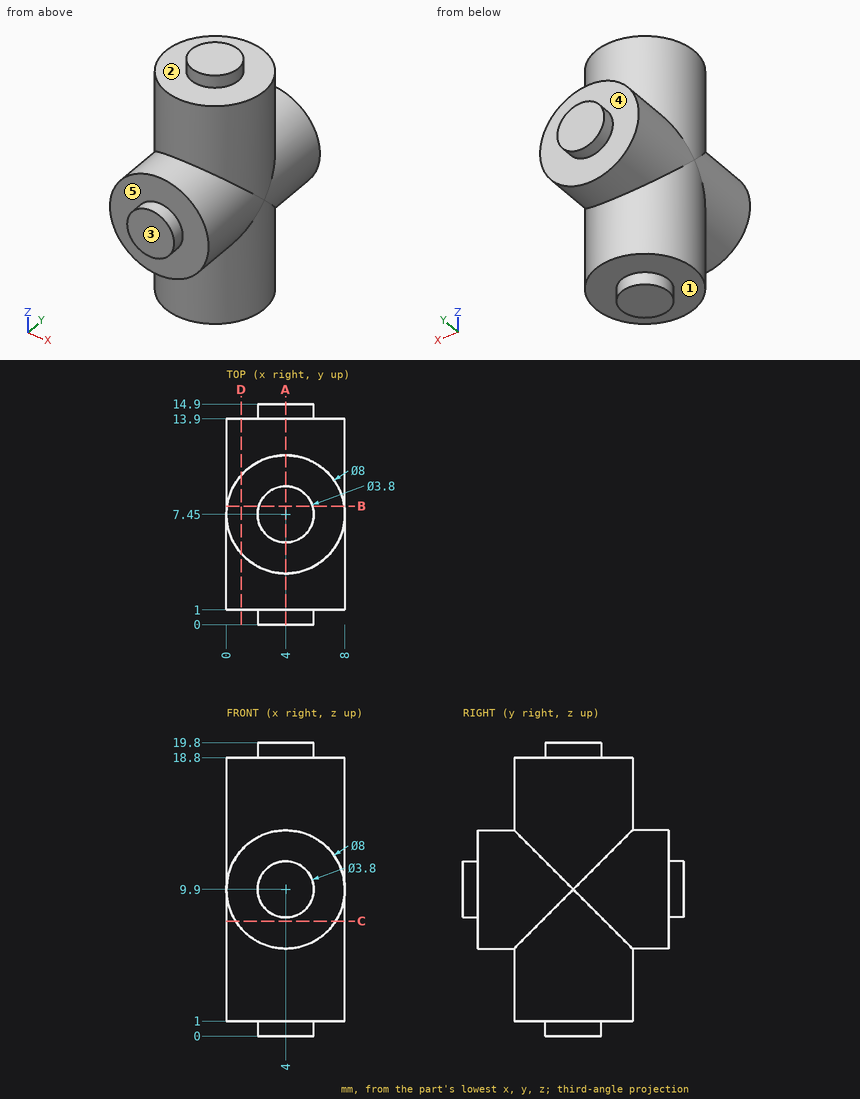
Could you check a few things on this drawing? It's one solid part, dimensions in mm from its lowest x, y, z. A direction names the side the tool comes from. Coordinates: 2 decimals unless noted, no trailing zeros. Order: outer loops, then holes, each group sorted by start corner. A loop starts at its lowest first (then second) coordinate and runs counter-clockwise, first axis right, second up. Notation, with made-up numbers: (-9, 28) - (13, 28) arc R24 cw to (13, 60) - close; hole circle Ø9 at (-12.75, 88). An arc over 180 degrees is marked (long way). Answer as a JSON object with one key per item and string values. Group by question number.
Q1. Imagine slicing it at A-A (x = 4). Please give me the cut outline in (y, z), and give its area (3 significant figures).
Q2. Imagine slicing it at B-B (y = 8). Please give me the cut outline in (x, z).
Q3. Imagine slicing it at D-D (x = 1). Please give me the cut outline in (y, z), and give its area (3 significant figures).
Q4. Imagine slicing it at C-C (z = 7.75). Please give me the cut outline in (x, y).
Q5. I need wall thicknesses on line 1 (Y direction, x = 2, z = 13); line 2 (Z direction, x = 7.25, y = 7.25); line 3 (Y direction, x = 4.25, z = 19). Which ranges of each line are inside material? Lowest first, please. Write a range as from..to.
Q6. On a 3-axis mill with a long thin cutter (end or side, diameter ignored), from which of +Z, -Z, +X, -X, +Y, -Y can I reach the whole of each face in a straight line? I mean the marked faces 1, 2, 3, 4 and 5. Say none if no direction works.
Q7. Will these pins go through, and if not, where does the flat tip stop? P1, Ø1, axis at x = 4, z = 16, coming from the -Y side; P2, Ø4, axis at x = 2.5, y = 13, coming from the +Z side; P3, Ø4, axis at y = 12, z = 17.5, coming from the -X side.
Determined:
{
 "1": {"outline": "(0, 8) - (1, 8) - (1, 5.9) - (3.45, 5.9) - (3.45, 1) - (5.55, 1) - (5.55, 0) - (9.35, 0) - (9.35, 1) - (11.45, 1) - (11.45, 5.9) - (13.9, 5.9) - (13.9, 8) - (14.9, 8) - (14.9, 11.8) - (13.9, 11.8) - (13.9, 13.9) - (11.45, 13.9) - (11.45, 18.8) - (9.35, 18.8) - (9.35, 19.8) - (5.55, 19.8) - (5.55, 18.8) - (3.45, 18.8) - (3.45, 13.9) - (1, 13.9) - (1, 11.8) - (0, 11.8) - close", "area": "197 mm2"},
 "2": {"outline": "(0.04, 1) - (2.18, 1) - (2.18, 0) - (5.82, 0) - (5.82, 1) - (7.96, 1) - (7.96, 9.35) arc R4 ccw to (7.96, 10.45) - (7.96, 18.8) - (5.82, 18.8) - (5.82, 19.8) - (2.18, 19.8) - (2.18, 18.8) - (0.04, 18.8) - (0.04, 10.45) arc R4 ccw to (0.04, 9.35) - close"},
 "3": {"outline": "(1, 7.25) - (4.8, 7.25) - (4.8, 1) - (10.1, 1) - (10.1, 7.25) - (13.9, 7.25) - (13.9, 12.55) - (10.1, 12.55) - (10.1, 18.8) - (4.8, 18.8) - (4.8, 12.55) - (1, 12.55) - close", "area": "134 mm2"},
 "4": {"outline": "(0.63, 1) - (7.37, 1) - (7.37, 5.3) arc R4 ccw to (7.37, 9.6) - (7.37, 13.9) - (0.63, 13.9) - (0.63, 9.6) arc R4 ccw to (0.63, 5.3) - close"},
 "5": {"line 1": "y = 1..13.9", "line 2": "z = 1..18.8", "line 3": "y = 5.57..9.33"},
 "6": {"face 1": "-Z", "face 2": "+Z", "face 3": "+Z, -Z, +X, -X, -Y", "face 4": "+Y", "face 5": "-Y"},
 "7": {"P1": "stops at y = 3.45", "P2": "stops at z = 18.8", "P3": "stops at x = 0.92"}
}
